Job drawing, mm, ordinate dimensions from the low corner. One solid piece. A direction names the side the tool comes from. Give positions to 0.01 mm unless a question says otherwise; leave off trailing zeros. Loops run counter-clockwise (first coordinate to the right, second up) from the corner with the lowest first, then second, coordinate; pieces in that order, holes last.
Item 1: Drop flat-ended pins along their axis: P1, Ø3, axis at x = 14, z = 15, coming from the -Y side; P2, Ø12, axis at y = 2.5, z = 12.5, coming from the +X side; P3, Ø6, axis at x = 16.5, z = 9.5, coming from the +Y side; P4, Ø3, axis at x = 4.5, y = 12, coming from the +Z side. Give the stop position or say it passes through.
Item 2: Mould opens along Y. For the marked faces 3, 4, 5 and 6 say: released by +Y, released by -Y, zero draft, split by the parting line, or undercut.
Item 3: Saw through at C-C on z = 9.5. Give the cut face in (x, y), plus the area to 3 significant figures.
Item 4: Probe probe 1 along Y at (x, z) = (10, 22); probe 2 along Y at (x, z) = (10, 38.25); probe 3 along Z at (x, y) = (10.5, 15.5). List the from-to ranges inside material, lowest first.
Item 5: Saw through at D-D on x = 15.5. Give the cut face in (y, z).
Item 6: Saw through at A-A on x = 10. Give the cut face in (y, z).
Item 7: Which spindle directions (+Z, -Z, +X, -X, +Y, -Y) get a long thin tool onto all of the face, cutting with end or side? Do the marked faces 1 and 2. Say none if no direction does.
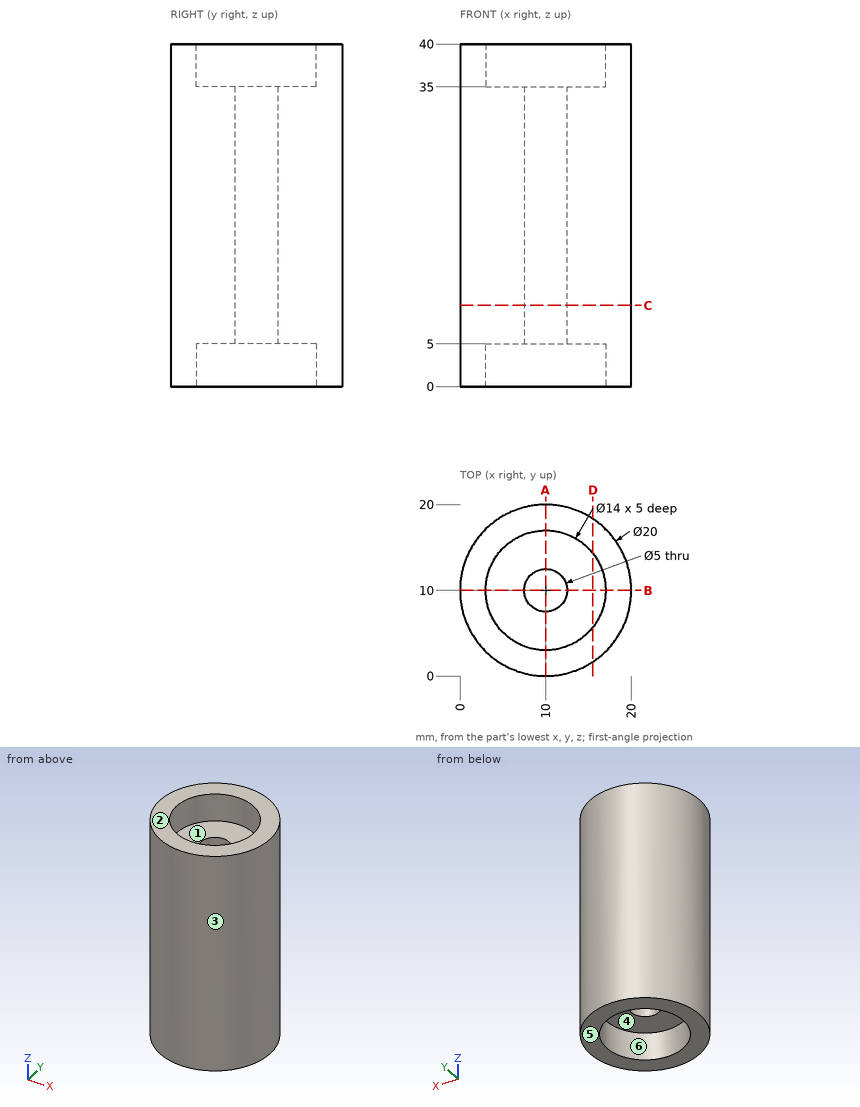
Results below:
1. P1: stops at y = 0.32
1. P2: stops at x = 19.89
1. P3: stops at y = 19.37
1. P4: stops at z = 40
2. face 3: split by the parting line
2. face 4: undercut
2. face 5: zero draft
2. face 6: undercut
3. outline: circle Ø20 at (10, 10); hole circle Ø5 at (10, 10)
3. area: 295 mm2
4. probe 1: y = 0 to 7.5, 12.5 to 20
4. probe 2: y = 0 to 3, 17 to 20
4. probe 3: z = 5 to 35
5. outline: (1.65, 0) - (5.67, 0) - (5.67, 5) - (14.33, 5) - (14.33, 0) - (18.35, 0) - (18.35, 40) - (14.33, 40) - (14.33, 35) - (5.67, 35) - (5.67, 40) - (1.65, 40) - close
6. outline: (0, 0) - (3, 0) - (3, 5) - (7.5, 5) - (7.5, 35) - (3, 35) - (3, 40) - (0, 40) - close; (12.5, 5) - (17, 5) - (17, 0) - (20, 0) - (20, 40) - (17, 40) - (17, 35) - (12.5, 35) - close
7. face 1: +Z
7. face 2: +Z, +X, -X, +Y, -Y
